Check sheet for the modelled part. Datum: model origin and axes. Units: mm. Face numbers are marked on the shaded views. Coordinates: 2 decimals unless noted, no trailing zeros. Loops run counter-clockwise (first coordinate to the right, second up) from the corner with the lowest first, then second, coordinate; pieces in that order, holes last. Notation, with made-up numbers: (78, 61.25) - (99, 61.25) arc R23 ccw to (99, 89.25) - close; hole circle Ø5 at (23, 79.5). An arc over 180 degrees is marked (long way). Answer as a JSON object with one key per item and string values. Group by question number.
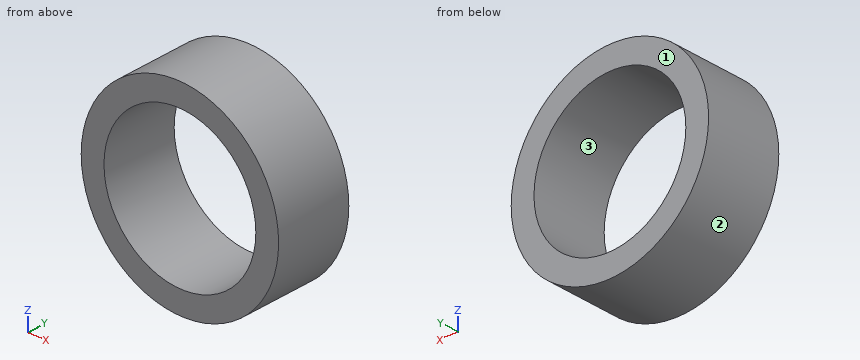
from build123d import *

# Parameters (mm, degrees)
CYLINDER005_R          = 5
CYLINDER005_DEPTH      = 5
CYLINDER005_ROLL_ANGLE = 90
CYLINDER006_R          = 6.5
CYLINDER006_DEPTH      = 5
CYLINDER006_ROLL_ANGLE = 90


with BuildPart() as cylinder005:
    # Cylinder005 → Cylinder005 (new body)
    with BuildSketch(Plane.XY):
        Circle(CYLINDER005_R)
    extrude(amount=CYLINDER005_DEPTH)


with BuildPart() as cylinder005_1:
    # Cylinder005 roll: moved
    add(cylinder005.part.rotate(Axis((0, 0, 0), (1, 0, 0)), CYLINDER005_ROLL_ANGLE))


with BuildPart() as cylinder005_2:
    # Cylinder005 placement: moved
    add(cylinder005_1.part.moved(Location((-5.4, 46, 0))))


with BuildPart() as cut001:
    # Cylinder006 → Cylinder006 (new body)
    with BuildSketch(Plane.XY):
        Circle(CYLINDER006_R)
    extrude(amount=CYLINDER006_DEPTH)


with BuildPart() as cut001_1:
    # Cylinder006 roll: moved
    add(cut001.part.rotate(Axis((0, 0, 0), (1, 0, 0)), CYLINDER006_ROLL_ANGLE))


with BuildPart() as cut001_2:
    # Cylinder006 placement: moved
    add(cut001_1.part.moved(Location((-5.4, 46, 0))))

    # Cut001: cut Cylinder005
    add(cylinder005_2.part, mode=Mode.SUBTRACT)


solid = cut001_2.part
1. Release check for a two-part mould opening along X. For the marked faces 1, 2 and 3 record: released by +X, released by -X, zero draft, split by the parting line, or undercut.
2. Sectioned sample at A-A on z = 0. Record the cut outline in (x, y).
3. Material ranges on line 1 (Z direction, x = -5.25, y = 45.4); line 2 (X direction, y = 42.5, z = 2.5); line 3 (Z direction, x = -10, y = 42.6), recorded low to high.
4. Sectioned sample at C-C on y = 44.1. Record the cut outline in (x, z).
5. Sectioned sample at D-D on z = -5.5. Record the cut outline in (x, y), plus the area to 3 significant figures.
6. Sectioned sample at B-B on x = -5.4. Record the cut outline in (y, z), plus the area to 3 significant figures.
Answers follow:
{
 "1": {"face 1": "zero draft", "face 2": "split by the parting line", "face 3": "undercut"},
 "2": {"outline": "(-11.9, 41) - (-10.4, 41) - (-10.4, 46) - (-11.9, 46) - close; (-0.4, 41) - (1.1, 41) - (1.1, 46) - (-0.4, 46) - close"},
 "3": {"line 1": "z = -6.5 to -5, 5 to 6.5", "line 2": "x = -11.4 to -9.73, -1.07 to 0.6", "line 3": "z = -4.59 to -1.96, 1.96 to 4.59"},
 "4": {"outline": "circle Ø13 at (-5.4, 0); hole circle Ø10 at (-5.4, 0)"},
 "5": {"outline": "(-8.86, 41) - (-1.94, 41) - (-1.94, 46) - (-8.86, 46) - close", "area": "34.6 mm^2"},
 "6": {"outline": "(41, -6.5) - (46, -6.5) - (46, -5) - (41, -5) - close; (41, 5) - (46, 5) - (46, 6.5) - (41, 6.5) - close", "area": "15.0 mm^2"}
}
